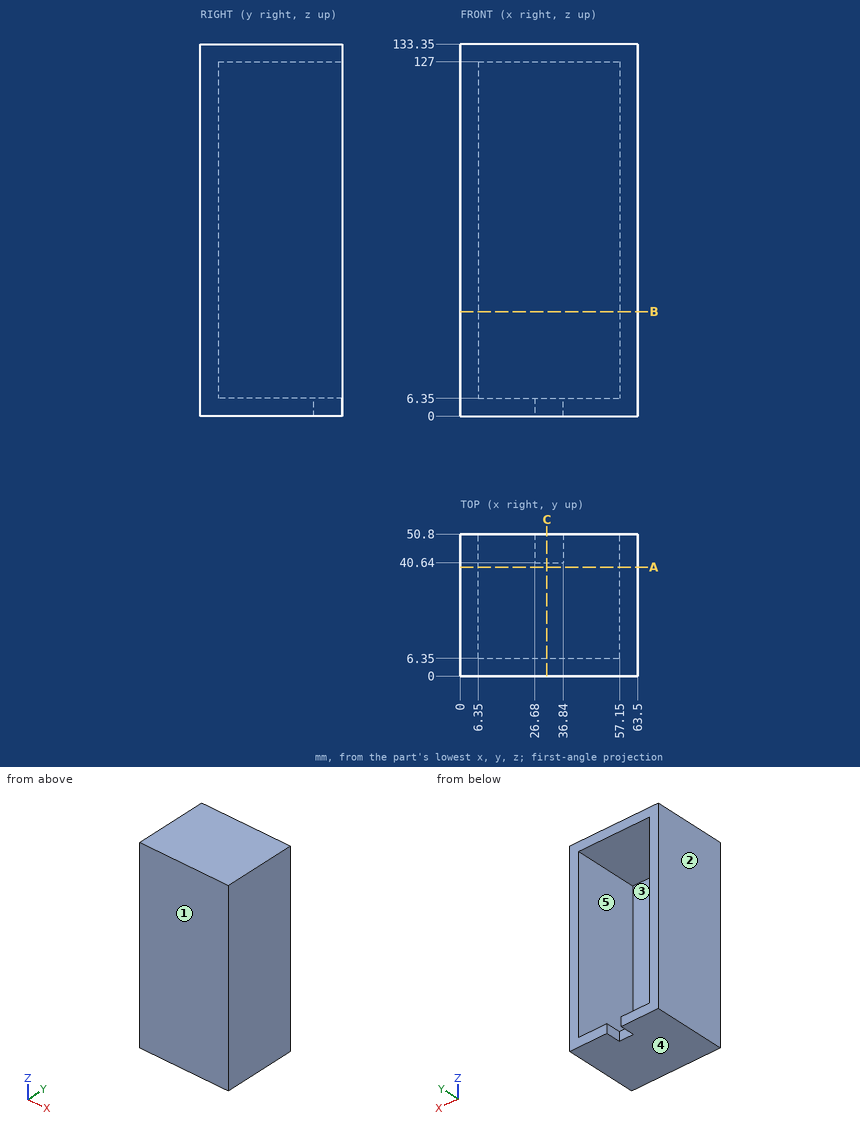
Source: three-view drawing plus pictorial views. Frame: mm from the lowest corner of the part. A direction names the side the tool comes from. Give positions to 0.01 mm unless a question says otherwise; leave off trailing zeros. Loops run counter-clockwise (first coordinate to the right, second up) from the corner with the lowest first, then second, coordinate; pieces in that order, holes last. Notation, with made-up numbers: (29.25, 41) -> (82.25, 41) arc R21 cw to (82.25, 62) -> close; hole circle Ø6 at (37, 68). An arc over 180 degrees is marked (long way). Use a Markdown table: item, result. Add a question column.
(1) Section query A-A (y = 39). Output: boundary loops of the cut face in (x, z).
(2) Section query C-C (x = 31). Output: boundary loops of the cut face in (y, z).
(3) Ray query, line 1 (X direction, y = 46, z = 50.5); line 2 (Z direction, x = 14, y = 30.5); line 3 (Y direction, x = 9.5, z = 19). Return the intervals inside material, ascending.
(4) Section query B-B (z = 37.5). Output: boundary loops of the cut face in (x, y), then the cut area to 3 significant figures.
(5) Access query for the marked faces 4 and 5. Directions: +Z, -Z, +X, -X, +Y, -Y. A direction counts if a zero-diameter tool reaches every point of the face in a straight line with its end or side. Return the directions, or none.
(6) Pull-direction query (X, two-part tool) for the marked faces 1, 2 and 3; classes: +X half, -X half, draft (parallel to the pull), parting line (faces both ways), or undercut.
(7) First-contact query: pin 1 Ø1.5 at (x, y) = (16, 17.5) entering from -Z; pin 2 Ø3 at (x, z) = (30, 2) entering from +Y; pin 3 Ø8 at (x, z) = (38.5, 24.5) entering from +Y. Flat tips, straight axial feed; report the tip coordinate or a pass-through.
Checked values:
| question | item | result |
|---|---|---|
| 1 | outline | (0, 0) -> (63.5, 0) -> (63.5, 133.35) -> (0, 133.35) -> close; hole (6.35, 6.35) -> (57.15, 6.35) -> (57.15, 127) -> (6.35, 127) -> close |
| 2 | outline | (0, 0) -> (40.64, 0) -> (40.64, 6.35) -> (6.35, 6.35) -> (6.35, 127) -> (50.8, 127) -> (50.8, 133.35) -> (0, 133.35) -> close |
| 3 | line 1 | 0 to 6.35, 57.15 to 63.5 |
| 3 | line 2 | 0 to 6.35, 127 to 133.35 |
| 3 | line 3 | 0 to 6.35 |
| 4 | outline | (0, 0) -> (63.5, 0) -> (63.5, 50.8) -> (57.15, 50.8) -> (57.15, 6.35) -> (6.35, 6.35) -> (6.35, 50.8) -> (0, 50.8) -> close |
| 4 | area | 968 mm^2 |
| 5 | face 4 | -Z, +X, -X, +Y, -Y |
| 5 | face 5 | +Y |
| 6 | face 1 | draft |
| 6 | face 2 | -X half |
| 6 | face 3 | undercut |
| 7 | pin 1 | z = 0 |
| 7 | pin 2 | y = 40.64 |
| 7 | pin 3 | y = 6.35 |
